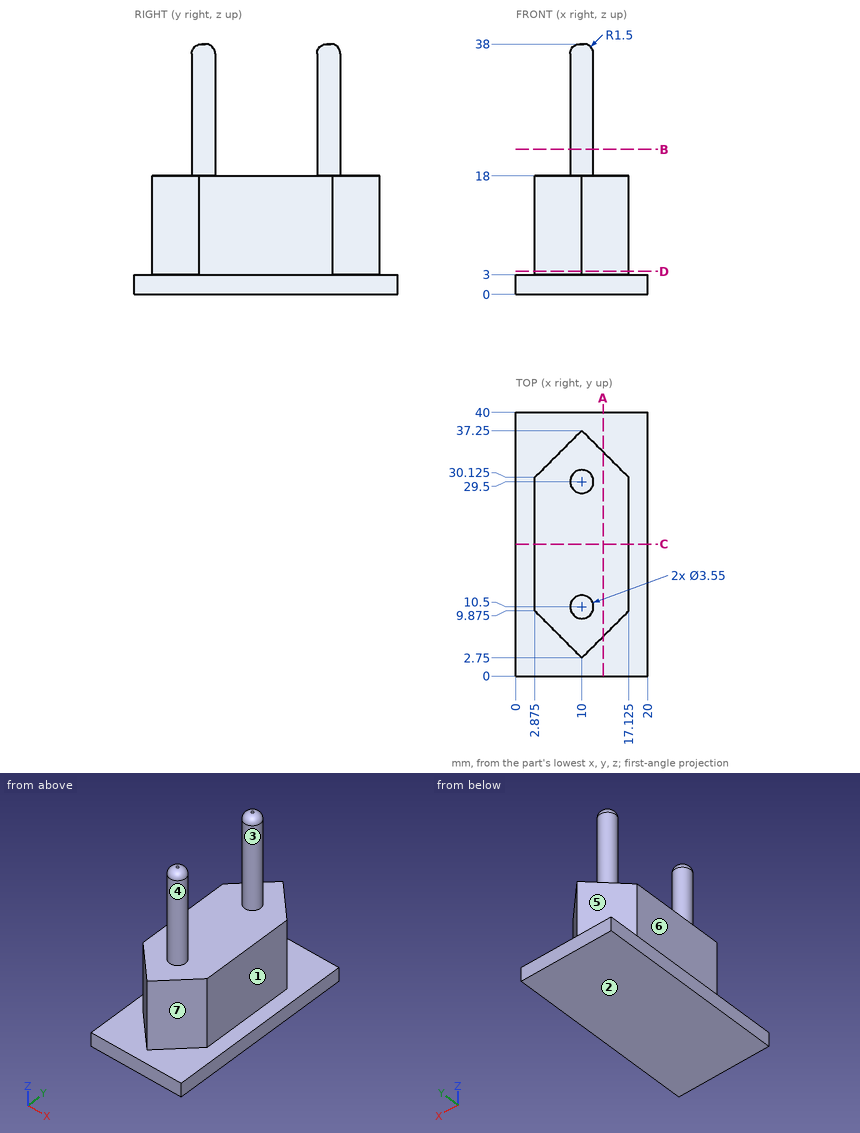
Here's the drawing with two shaded views (mm, measured from the low corner). I have some questions. A direction names the side the tool comes from. Coordinates: 2 decimals unless noted, no trailing zeros. Loops run counter-clockwise (first coordinate to the right, second up) from the corner with the lowest first, then second, coordinate; pieces in that order, holes last. Notation, with made-up numbers: (88, 38) -> (98, 38) arc R31 cw to (98, 74) -> close; hole circle Ø9 at (50, 4). An arc over 180 degrees is marked (long way). Answer as a JSON object with one key per item and string values.
1) Imagine slicing it at B-B (z = 22). Please give me the cut outline in (x, y) (3 decimals), then the cut area to 3 significant figures.
Results:
{"outline": "circle Ø3.55 at (10, 10.5); circle Ø3.55 at (10, 29.5)", "area": "19.8 mm^2"}
2) For P1, Ø6, axis at x = 5.5, z = 16.5, coming from the -Y side; P2, Ø12, axis at x = 12, z = 15.5, coming from the -Y side; P3, Ø8, axis at x = 15, z = 16, coming from the +Y side; P4, Ø11.5, axis at x = 10.5, y = 16.5, coming from the +Z side, each with a flat end and sliding along its axis, tell me the tip position at first contact or that it passes through.
Results:
{"P1": "stops at y = 4.25", "P2": "stops at y = 2.75", "P3": "stops at y = 36.25", "P4": "stops at z = 38"}
3) Imagine slicing it at D-D (z = 3.5). Please give me the cut outline in (x, y) (3 decimals), then the cut area to 3 significant figures.
Results:
{"outline": "(2.875, 9.875) -> (10, 2.75) -> (17.125, 9.875) -> (17.125, 30.125) -> (10, 37.25) -> (2.875, 30.125) -> close", "area": "390 mm^2"}
4) For the marked faces 1, 2 and 3, which set-ups out of +Z, -Z, +X, -X, +Y, -Y let a thin tool reach every point of the face, with its end or its side?
Results:
{"face 1": "+Z, +X, +Y, -Y", "face 2": "-Z, +X, -X, +Y, -Y", "face 3": "+Z"}
5) Thinking about a two-plate mould opening in Y: for the marked faces 4, 5, 6 and 7, which applies, pulls with the +Y half, pulls with the -Y half, needs draft (parallel to the pull), parting line crosses it, or undercut?
Results:
{"face 4": "undercut", "face 5": "pulls with the +Y half", "face 6": "needs draft", "face 7": "pulls with the -Y half"}
6) Imagine slicing it at C-C (y = 20). Please give me the cut outline in (x, z) (3 decimals).
Results:
{"outline": "(0, 0) -> (20, 0) -> (20, 3) -> (17.125, 3) -> (17.125, 18) -> (2.875, 18) -> (2.875, 3) -> (0, 3) -> close"}
7) If I drill on line 1 (Z direction, x = 11, y = 25.5); line 2 (X direction, y = 29, z = 10.5) (3 decimals); line 3 (Z direction, x = 8, y = 36), over which ranges is the centre line in solid material (lowest first)?
Results:
{"line 1": "z = 0 to 18", "line 2": "x = 2.875 to 17.125", "line 3": "z = 0 to 3"}
8) Imagine slicing it at A-A (x = 13.25). Please give me the cut outline in (y, z).
Results:
{"outline": "(0, 0) -> (40, 0) -> (40, 3) -> (34, 3) -> (34, 18) -> (6, 18) -> (6, 3) -> (0, 3) -> close"}
